Geometry: final body of the model. Coordinates: model frame, mm. Give positions to 0.01 mm unless a question says otherwise; leave off trailing zeros. Write each loop counter-clockwise with the first axis right and the second up, starting at its lowest first coordinate (ties: lowest second). Pieces come first, ordered by that corner, then holes.
Q1. Section B-B (y = -12). Return the cut outline in (x, z), plus the area to 3 significant figures.
Q2. Pin query (flat end, axial travel): pin 1 Ø1 at (x, z) = (-40.5, 3) entering from +Y; pin 2 Ø1.5 at (x, z) = (120, 4.5) entering from +Y; pin 3 Ø2 at (x, y) = (-37, 154.5) entering from -Z; pin 4 Ø2 at (y, z) = (-90, 4) entering from +X. Return the tip coordinate at first contact, or that it passes through.
Q3. Section D-D (x = -68.5). Return the cut outline in (y, z), plus the area to 3 significant figures.
Q4. Line query: line 1 (Y direction, x = 0, z = 1.95); line 2 (Y direction, x = 80, z = 1.95); line 3 (X direction, y = 165.5, z = 3.15). Output: solid intervals per line, ascending.
Q5. Section A-A (x = 0). Return the cut outline in (y, z), plus the area to 3 significant figures.
Q6. Section C-C (z = 1.4). Return the cut outline in (x, y).
from build123d import *

# Parameters (mm, degrees)
F0_R     = 222.5
F0_R_2   = 20
F1_DEPTH = 5


with BuildPart() as f1:
    # F0 (on Top) → F1 (new body)
    with BuildSketch(Plane.XY):
        Circle(F0_R)
        with Locations((-138.564065, -80)):
            Circle(F0_R_2, mode=Mode.SUBTRACT)
        with Locations((138.564065, -80)):
            Circle(F0_R_2, mode=Mode.SUBTRACT)
        with BuildLine():
            ThreePointArc((7, 119.795659), (87.292611, 82.340755), (120, 0))
            ThreePointArc((120, 0), (87.292611, -82.340755), (7, -119.795659))
            Line((7, -119.795659), (7, -125))
            Line((7, -125), (-7, -125))
            Line((-7, -125), (-7, -119.795659))
            ThreePointArc((-7, -119.795659), (-120, 0), (-7, 119.795659))
            Line((-7, 119.795659), (-7, 125))
            Line((-7, 125), (7, 125))
            Line((7, 125), (7, 119.795659))
        make_face(mode=Mode.SUBTRACT)
        with Locations((0, 160)):
            Circle(F0_R_2, mode=Mode.SUBTRACT)
    extrude(amount=F1_DEPTH)


solid = f1.part
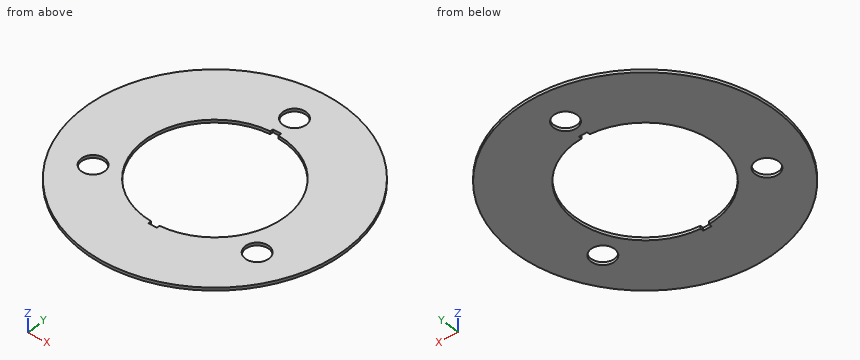
Computed:
1. outline: (-222.18, 0) - (-119.4, 0) - (-119.4, 5) - (-222.18, 5) - close; (119.4, 0) - (222.18, 0) - (222.18, 5) - (119.4, 5) - close
1. area: 1,030 mm2
2. pin 1: stops at y = 218.87
2. pin 2: stops at y = 187.84
2. pin 3: stops at z = 0
2. pin 4: stops at x = 203.92
3. outline: (-211.69, 0) - (-98.53, 0) - (-98.53, 5) - (-211.69, 5) - close; (98.53, 0) - (211.69, 0) - (211.69, 5) - (98.53, 5) - close
3. area: 1,130 mm2
4. line 1: y = -222.5 to -125, 125 to 140, 180 to 222.5
4. line 2: y = -207.62 to -89.44, 89.44 to 207.62
4. line 3: x = -148.71 to -19.23, 19.23 to 148.71
5. outline: (-222.5, 0) - (-125, 0) - (-125, 5) - (-222.5, 5) - close; (125, 0) - (140, 0) - (140, 5) - (125, 5) - close; (180, 0) - (222.5, 0) - (222.5, 5) - (180, 5) - close
5. area: 775 mm2
6. outline: circle Ø445 at (0, 0); hole circle Ø40 at (-138.56, -80); hole circle Ø40 at (0, 160); hole (-7, -125) - (7, -125) - (7, -119.8) arc R120 ccw to (120, 0) arc R120 ccw to (7, 119.8) - (7, 125) - (-7, 125) - (-7, 119.8) arc R120 ccw to (-7, -119.8) - close; hole circle Ø40 at (138.56, -80)
